Input: part model. Units: mm. Frame: model coordinates. A direction names the side the tool comes from. Coordinates: 2 decimals unless noted, no trailing zeros. Write each loop counter-clockwise with the first axis right and the second up, starting at its lowest first coordinate (ties: lowest second). Pieces come first, ordered by that corner, then holes. Notation, with made-up numbers: M 45.5,62 L 85.5,62 A32 ccw 85.5,88 Z; hole C -16.75,-25.75 d5. An arc over 180 degrees is marked long. Use one line per item in the form item = value.
from build123d import *

# Parameters (mm, degrees)
SKETCH_1_W          = 150
SKETCH_1_H          = 125
EXTRUDE_1_DEPTH     = 15
SKETCH_2_W          = 150
SKETCH_2_H          = 40
EXTRUDE_2_DEPTH     = 70
SKETCH_3_W          = 136
SKETCH_3_H          = 26
CUT_EXTRUDE_1_DEPTH = 130.44593466
SKETCH_4_R          = 8
CUT_EXTRUDE_2_DEPTH = 121.130137767
RIB_1_REACH         = 131.446
SKETCH_5_WALL_W     = 342.78356609
SKETCH_5_WALL_H     = 20
CUT_EXTRUDE1_REACH  = 185.388


with BuildPart() as part:
    # Эскиз1 → Бобышка-Вытянуть1 (new body)
    with BuildSketch(Plane.XY):
        Rectangle(SKETCH_1_W, SKETCH_1_H)
    extrude(amount=EXTRUDE_1_DEPTH)

    # Эскиз2 → Бобышка-Вытянуть2 (add)
    with BuildSketch(Plane.XY.offset(15)):
        Rectangle(SKETCH_2_W, SKETCH_2_H)
    extrude(amount=EXTRUDE_2_DEPTH)

    # Эскиз3 → Вырез-Вытянуть1 (cut, through all)
    with BuildSketch(Plane.XY.offset(85)):
        Rectangle(SKETCH_3_W, SKETCH_3_H)
    extrude(amount=-CUT_EXTRUDE_1_DEPTH, mode=Mode.SUBTRACT)

    # Эскиз4 → Вырез-Вытянуть2 (cut, through all)
    with BuildSketch(Plane.XY.offset(15)):
        with BuildLine():
            Line((48, 62.5), (48, 47.5))
            ThreePointArc((48, 47.5), (54.5, 41), (61, 47.5))
            Line((61, 47.5), (61, 62.5))
            Line((61, 62.5), (48, 62.5))
        make_face()
        with Locations((45, -47.5)):
            Circle(SKETCH_4_R)
    cut_extrude_2 = extrude(amount=-CUT_EXTRUDE_2_DEPTH, mode=Mode.SUBTRACT)

    # Эскиз5 wall → Ребро1 (add, up to next)
    with BuildSketch(Plane(origin=(0, -41.25, 50), x_dir=(0, -0.518978134242, -0.854787515222), z_dir=(0, 0.854787515222, -0.518978134242)), mode=Mode.PRIVATE) as rib_1_sk1:
        Rectangle(SKETCH_5_WALL_W, SKETCH_5_WALL_H)
    rib_1_tool1 = extrude(rib_1_sk1.sketch, amount=RIB_1_REACH, mode=Mode.PRIVATE) - part.part
    add(rib_1_tool1.solids().sort_by_distance((0, -41.25, 50))[0])

    # Зеркальное отражение1: Вырез-Вытянуть2 across plane
    add(cut_extrude_2.mirror(Plane(origin=(0, 0, 0), x_dir=(0, 0, 1), z_dir=(1, 0, 0))), mode=Mode.SUBTRACT)

    # Sketch1 → Cut-Extrude1 (cut, up to next)
    with BuildSketch(Plane(origin=(75, 0, 0), x_dir=(0, 0, -1), z_dir=(1, 0, 0)), mode=Mode.PRIVATE) as cut_extrude1_sk1:
        with BuildLine():
            Line((-85, 7.5), (-60, 7.5))
            ThreePointArc((-60, 7.5), (-52.5, 0), (-60, -7.5))
            Line((-60, -7.5), (-85, -7.5))
            ThreePointArc((-85, -7.5), (-92.5, 0), (-85, 7.5))
        make_face()
    cut_extrude1_tool1 = extrude(cut_extrude1_sk1.sketch, amount=-CUT_EXTRUDE1_REACH, mode=Mode.PRIVATE) & part.part
    add(cut_extrude1_tool1.solids().sort_by_distance((75, 0, 72.5))[0], mode=Mode.SUBTRACT)


solid = part.part
(1) Section query A-A on x = 25.5. Return the cut outline in (y, z).
Computed:
outline = M -62.5,0 L -13,0 L -13,85 L -20,85 L -20,15 L -62.5,15 Z; M 13,0 L 62.5,0 L 62.5,15 L 20,15 L 20,85 L 13,85 Z
(2) First-contact query: pin 1 Ø13 at (x, y) = (-7, 31.5) entering from +Z; pin 2 Ø2 at (y, z) = (-46, 35) entering from -X; pin 3 Ø7.5 at (x, z) = (72.5, 69) entering from +Y. Flat tips, straight axial feed; report the tip coordinate or a pass-through.
Computed:
pin_1 = 15
pin_2 = -10
pin_3 = 20
(3) Line query: probe 1 along X at (y, z) = (-47, 5); probe 2 along Y at (x, z) = (45, 4.5); probe 3 along X at (y, z) = (49, 11). Output: solid intervals per line, ascending.
Computed:
probe_1 = -75 to -52.98, -37.02 to 37.02, 52.98 to 75
probe_2 = -62.5 to -55.5, -39.5 to -13, 13 to 62.5
probe_3 = -75 to -61, -48 to 48, 61 to 75
(4) Pull-direction query (Y, two-part tool) for faces 4 (the flat face through (-1, 62.5, 7)), 5 (the flat face through (-1, 42, 15)), 6 (the cylindrical face through (-39.1, -42.1, 7.6)); classes: pulls with the +Y half, pulls with the -Y half, needs draft (parallel to the pull), parting line crosses it, or undercut.
Computed:
face_4 = pulls with the +Y half
face_5 = needs draft
face_6 = undercut
(5) Section query D-D on y = -29.5. Return the cut outline in (x, z), plus the area to 3 significant figures.
Computed:
outline = M -75,0 L 75,0 L 75,15 L 10,15 L 10,69.35 L -10,69.35 L -10,15 L -75,15 Z
area = 3,340 mm^2
(6) Set-up query: faces 1 (the flat face through (61, 55, 8)), 2 (the cylindrical face through (71.55, 0.16, 52.5)), 3 (the flat face through (42, -20, 50)). Return all of +Z, -Z, +X, -X, +Y, -Y with unobstructed straight access to the full face (end or side cutting, diameter ignored); none if empty.
Computed:
face_1 = +Z, -Z, +Y
face_2 = +Z, +X
face_3 = +Z, +X, -Y
(7) Section query B-B on z = 49. Return the cut outline in (x, y), plus the area to 3 significant figures.
Computed:
outline = M -75,-20 L -10,-20 L -10,-41.86 L 10,-41.86 L 10,-20 L 75,-20 L 75,20 L -75,20 Z; hole M -68,-13 L 68,-13 L 68,13 L -68,13 Z
area = 2,900 mm^2
(8) Section query C-C on x = -45. Return the cut outline in (y, z).
Computed:
outline = M -62.5,0 L -55.5,0 L -55.5,15 L -62.5,15 Z; M -39.5,0 L -13,0 L -13,85 L -20,85 L -20,15 L -39.5,15 Z; M 13,0 L 62.5,0 L 62.5,15 L 20,15 L 20,85 L 13,85 Z
